Source: CAD feature listing. Evaluate the final solid. Frame: model axes, mm. A direction names the side the tool comes from. Give positions to 0.01 mm unless a question says otherwise; leave off trailing zeros. Loops run counter-clockwise (first coordinate to the right, second up) from the corner with the lowest first, then second, coordinate; pieces in that order, holes last. Notation, with made-up numbers: M 0,72 L 59,72 A25 cw 59,95 Z; hole C 44.5,38.5 d11. An arc over 180 degrees is marked long. Answer in a Markdown table with one row per item.
```python
from build123d import *

# Parameters (mm, degrees)
F0_W     = 203.2
F0_H     = 31
F1_DEPTH = 3
F3_DEPTH = 203.2
F4_T     = -2.54


with BuildPart() as f1:
    # F0 (on Front) → F1 (new body)
    with BuildSketch(Plane.XZ):
        with Locations((-101.6, 15.5)):
            Rectangle(F0_W, F0_H)
    extrude(amount=F1_DEPTH)

    # F2 (on face) → F3 (join)
    with BuildSketch(Plane.YZ):
        Polygon((0, 31), (0, 0), (17.857041, 6.635404), align=None)
    extrude(amount=-F3_DEPTH)

    # F4
    f4_openings = [f1.faces().sort_by_distance(p)[0] for p in [
        (-101.6, 8.928521, 18.817702),
    ]]
    offset(amount=F4_T, openings=f4_openings)


solid = f1.part
```
Q1. Section query C-C (y = 7.5). Output: boundary loops of the cut face in (x, z).
Values follow:
| item | result |
|---|---|
| outline | M -203.2,2.79 L 0,2.79 L 0,20.77 L -2.54,20.77 L -2.54,5.5 L -200.66,5.5 L -200.66,20.77 L -203.2,20.77 Z |
Q2. Ray query, probe 1 along X at (y, z) = (5.75, 9); probe 2 along Y at (x, z) = (-60.5, 16); probe 3 along Z at (x, y) = (-174.5, 0.5). Return the intervals inside material, ascending. Write a range as from..to.
Values follow:
| item | result |
|---|---|
| probe 1 | -203.2..-200.66, -2.54..0 |
| probe 2 | -3..-0.46 |
| probe 3 | 0.19..2.9, 28.46..30.32 |
Q3. Mould query, pull axis Y, two halves, no side actions, for faces 1 (the flat face through (-200.66, 6, 13)), 2 (the flat face through (-103, -3, 16)), 3 (the flat face through (-100.18, 8.8, 3.27)). Classes: +Y half, -Y half, draft (parallel to the pull), parting line (faces both ways), or undercut.
Values follow:
| item | result |
|---|---|
| face 1 | undercut |
| face 2 | -Y half |
| face 3 | +Y half |
Q4. Reachability of faces 4 (the flat face through (-101.126, 1.695, 28.687)), 5 (the flat face through (-2.54, 6, 13)) from +Z, -Z, +X, -X, +Y, -Y: full face, straight path, thin tool, end or side. Return the list, or none.
Values follow:
| item | result |
|---|---|
| face 4 | +Z, +X, -X, +Y |
| face 5 | none |
Q5. Contact query for flat-ended pins moving along their axis: pin 1 Ø5 at (x, y) = (-172, 6.5) entering from -Z; pin 2 Ø0.7 at (x, y) = (-74.5, 1) entering from -Z; pin 3 Ø1 at (y, z) = (9, 19.5) entering from +X; pin 4 Ø5 at (x, y) = (-90.5, 15) entering from -Z. Output: stop coordinate, or through.
Values follow:
| item | result |
|---|---|
| pin 1 | z = 1.49 |
| pin 2 | z = 0.24 |
| pin 3 | x = 0 |
| pin 4 | z = 4.64 |
Q6. Section query B-B (z = 12). Output: boundary loops of the cut face in (x, y).
Values follow:
| item | result |
|---|---|
| outline | M -203.2,-3 L 0,-3 L 0,13.93 L -2.54,13.93 L -2.54,-0.46 L -200.66,-0.46 L -200.66,13.93 L -203.2,13.93 Z |
